Autodesk Inventor part; units mm, degrees
ref_plane "Work Plane1" through (83.5, 0, -139.5) normal (1, 0, 0) x (0, 0, -1)
ref_plane "YZ Plane" through (0, 0, 0) normal (1, 0, 0) x (0, 1, 0)
ref_plane "XZ Plane" through (0, 0, 0) normal (0, 1, 0) x (-1, 0, 0)
sketch "Sketch1" plane through (0, 0, 0) normal (0, 1, 0) x (-1, 0, 0)
  line L0 (-83.5, 139.5) -> (83.5, 139.5)
  line L1 (83.5, 139.5) -> (83.5, -139.5)
  line L2 (83.5, -139.5) -> (-83.5, -139.5)
  line L3 (-83.5, -139.5) -> (-83.5, 139.5)
  line L4 (-83.5, 139.5) -> (83.5, -139.5) construction
  line L5 (83.5, 139.5) -> (-83.5, -139.5) construction
  point P0 (0, 0)
  dimension "d0" = 167
  dimension "d1" = 279
extrude "Extrusion1" add sketch "Sketch1" along normal blind 13.4
sketch "Sketch2" plane through (0, 13.4, 0) normal (0, 1, 0) x (1, 0, 0)
  line L0 (72.25, -115.05) -> (-72.25, -115.05)
  line L1 (-72.25, -115.05) -> (-72.25, 115.05)
  line L2 (-72.25, 115.05) -> (72.25, 115.05)
  line L3 (72.25, 115.05) -> (72.25, -115.05)
  line L4 (72.25, -115.05) -> (-72.25, 115.05) construction
  line L5 (-72.25, -115.05) -> (72.25, 115.05) construction
  point P0 (0, 0)
  dimension "d4" = 144.5
  dimension "d5" = 230.1
extrude "Extrusion2" cut sketch "Sketch2" against normal blind 8.4
sketch "Sketch4" plane through (0, 13.4, 0) normal (0, 1, 0) x (1, 0, 0)
  circle A0 centre (-77.5, -133.5) radius 1.25
  line L0 (-83.5, 139.5) -> (-83.5, -139.5)
  line L1 (-83.5, -139.5) -> (83.5, -139.5)
  circle A1 centre (-77.5, 133.5) radius 1.25
  line L2 (83.5, 139.5) -> (-83.5, 139.5)
  circle A2 centre (77.5, 133.5) radius 1.25
  line L3 (83.5, -139.5) -> (83.5, 139.5)
  circle A3 centre (77.5, -133.5) radius 1.25
  point P0 (0, 0)
  dimension "d16" = 2.5
  dimension "d17" = 6
  dimension "d18" = 6
  dimension "d19" = 2.5
  dimension "d20" = 6
  dimension "d21" = 6
  dimension "d22" = 2.5
  dimension "d23" = 6
  dimension "d24" = 6
  dimension "d25" = 2.5
  dimension "d26" = 6
  dimension "d27" = 6
extrude "Extrusion4" cut sketch "Sketch4" against normal through all contours A0 | A1 | A2 | A3
sketch "Sketch5" plane through (0, 13.4, 0) normal (0, 1, 0) x (1, 0, 0)
  line L0 (-72.25, -115.05) -> (-72.25, 115.05)
  line L1 (72.25, -115.05) -> (-72.25, -115.05)
  line L2 (-77.25, -120.05) -> (-72.25, -120.05)
  line L3 (-72.25, -120.05) -> (-72.25, 120.05)
  line L4 (-72.25, 120.05) -> (-77.25, 120.05)
  line L5 (-77.25, 120.05) -> (-77.25, -120.05)
  line L6 (72.25, 115.05) -> (72.25, -115.05)
  line L7 (77.25, -120.05) -> (72.25, -120.05)
  line L8 (72.25, -120.05) -> (72.25, 120.05)
  line L9 (72.25, 120.05) -> (77.25, 120.05)
  line L10 (77.25, 120.05) -> (77.25, -120.05)
  line L11 (-72.25, 115.05) -> (72.25, 115.05)
  line L12 (72.25, 120.05) -> (-72.25, 120.05)
  line L13 (-72.25, 120.05) -> (-72.25, 115.05)
  line L14 (-72.25, 115.05) -> (72.25, 115.05)
  line L15 (72.25, 115.05) -> (72.25, 120.05)
  line L16 (-72.25, -115.05) -> (72.25, -115.05)
  line L17 (72.25, -115.05) -> (72.25, -120.05)
  line L18 (72.25, -120.05) -> (-72.25, -120.05)
  line L19 (-72.25, -120.05) -> (-72.25, -115.05)
  point P0 (0, 0)
  dimension "d30" = 5
  dimension "d31" = 5
  dimension "d32" = 240.1
  dimension "d33" = 5
  dimension "d34" = 5
  dimension "d35" = 240.1
extrude "Extrusion5" add sketch "Sketch5" along normal blind 10 contours L3 L2 L5 L4 L0 | L1 L8 L18 L3 | L3 L12 L8 L11 | L6 L8 L9 L10 L7
sketch "Sketch7" plane through (0, 0, 0) normal (0, -1, 0) x (1, 0, 0)
  circle A0 centre (-77.5, -133.5) radius 1.25
  circle A1 centre (-77.5, -133.5) radius 1.75
  circle A2 centre (-77.5, 133.5) radius 1.25
  circle A3 centre (-77.5, 133.5) radius 1.75
  circle A4 centre (77.5, 133.5) radius 1.25
  circle A5 centre (77.5, 133.5) radius 1.75
  circle A6 centre (77.5, -133.5) radius 1.25
  circle A7 centre (77.5, -133.5) radius 1.75
  point P0 (0, 0)
  dimension "d42" = 3.5
  dimension "d43" = 3.5
  dimension "d44" = 3.5
  dimension "d45" = 3.5
extrude "Extrusion6" cut sketch "Sketch7" against normal blind 11.4 contours A0 | A1 | A2 | A3 | A4 | A5 | A7
sketch "Sketch8" plane through (83.5, 0, 139.5) normal (1, 0, 0) x (0, 0, -1)
  line L0 (139.5, 0) -> (139.5, 13.4)
  line L1 (0, 13.4) -> (279, 13.4)
sketch "Sketch9" plane through (0, 13.4, 0) normal (0, 1, 0) x (1, 0, 0)
  line L0 (83.5, -139.5) -> (83.5, 139.5)
  line L1 (83.5, 0) -> (77.25, 0)
  line L2 (77.25, 120.05) -> (77.25, -120.05)
  point P0 (0, 0)
sketch "Sketch10" plane through (77.25, 13.4, 120.05) normal (1, 0, 0) x (0, 0, -1)
  line L0 (-19.45, 0) -> (259.55, 0)
  line L1 (120.05, 0) -> (120.05, 10)
  line L2 (0, 10) -> (240.1, 10)
  point P0 (120.05, -13.4)
split_face "Split1"
split_face "Split2"
split_face "Split3"
ref_plane "Work Plane1" through (83.5, 0, -139.5) normal (1, 0, 0) x (0, 0, -1)
sketch "Sketch11" plane through (83.5, 0, -139.5) normal (1, 0, 0) x (0, 0, -1)
  line L0 (0, 0) -> (0, 13.4)
  line L1 (-139.5, 5) -> (-139.5, 23.4)
  line L2 (0, 0) -> (-139.5, 0)
  line L3 (-139.5, 0) -> (-139.5, 23.4)
  line L4 (-139.5, 23.4) -> (0, 23.4)
  line L5 (0, 23.4) -> (0, 0)
  point P0 (-139.5, 0)
extrude "Extrusion7" cut sketch "Sketch11" against normal blind 167.1625
sketch "Sketch12" plane through (83.5, 0, 0) normal (0, 0, -1) x (-1, 0, 0)
  line L0 (0, 0) -> (0, 13.4)
  circle A0 centre (5.625, 6.7) radius 2.375
  line L1 (167, 0) -> (167, 13.4)
  circle A1 centre (161.375, 6.7) radius 2.375
  line L2 (11.25, 5) -> (155.75, 5)
  circle A2 centre (58.5, 2.5) radius 1.375
  circle A3 centre (33.5, 2.5) radius 1.375
  circle A4 centre (108.5, 2.5) radius 1.375
  circle A5 centre (133.5, 2.5) radius 1.375
  point P0 (83.5, 0)
  dimension "d51" = 4.75
  dimension "d53" = 4.75
  dimension "d55" = 2.75
  dimension "d57" = 2.75
  dimension "d59" = 2.75
  dimension "d61" = 2.75
extrude "Extrusion8" add sketch "Sketch12" along normal blind 15
properties part number "Enclosure 2 Bottom" material "ABS Plastic"
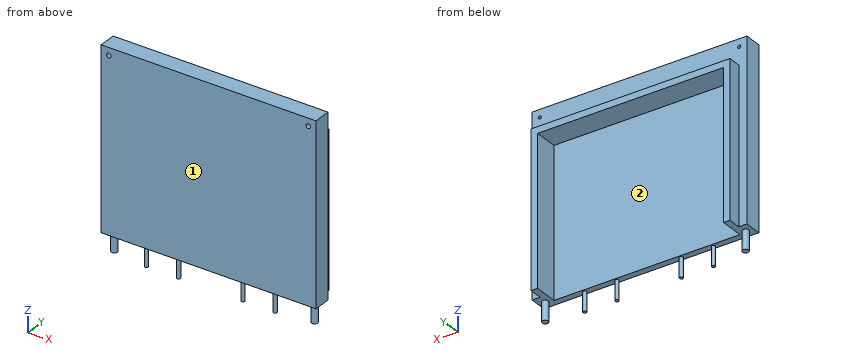
Design review of the part built by this model. Coordinates are the model's own, in mm. Face numbers are marked on the shaded views. Round coordinates to 2 decimals unless told otherwise and drop trailing zeros. Order: outer loops, then holes, each group sorted by start corner. A loop starts at its lowest first (then second) coordinate and runs counter-clockwise, first axis right, second up. Notation, with made-up numbers: M 81.5,32.25 L 119.5,32.25 A12 cw 119.5,51.25 Z; hole C 21,26 d1. An arc over 180 degrees is marked long. Answer as CSV lines item,"result". Start each with the question number.
1) Wall thickness on line 1 along X through (y, z) = (6, 133.5); line 2 along X through (y, z) = (11.9, 133.5); line 3 along X through (y, z) = (12.5, 73): over which ranges is each line inside the solid? List them lowest first. Write a range as [from, to].
2) The part is to be moulded in two halves that separate along X. For the marked faces 1 and 2, say which applies: +X half, -X half, draft (parallel to the pull), parting line (faces both ways), or undercut.
3) Add section A-A (z = -4). Give the boundary of the cut face in (x, y) (3 decimals).
4) Add section B-B (x = 68). Give the boundary of the cut face in (y, z), then the cut area to 3 significant figures.
5) Add section C-C (y = 15.25). Give the boundary of the cut face in (x, z).
6) Add section D-D (z = 91). Give the boundary of the cut face in (x, y).
7) For pin 1 Ø8 at (y, z) = (19, 72.5) entering from +X; pin 2 Ø6 at (x, z) = (-60, 22) entering from +Y; pin 3 Ø3 at (x, y) = (-32.5, 18) entering from +Z, all flat-tipped, find the tip position at first contact; note any pin that passes through.
Resolved:
1,line 1,"[-83.5, -79.25], [-75.75, 75.75], [79.25, 83.5]"
1,line 2,"[-83.5, -78.75], [-76.25, 76.25], [78.75, 83.5]"
1,line 3,"[-83.5, -72.25], [72.25, 83.5]"
2,face 1,"draft"
2,face 2,"undercut"
3,outline,"C -77.875,6.7 d4.75; C -50,2.5 d2.75; C -25,2.5 d2.75; C 25,2.5 d2.75; C 50,2.5 d2.75; C 77.875,6.7 d4.75"
4,outline,"M 0,0 L 5,0 L 5,115.05 L 23.4,115.05 L 23.4,120.05 L 13.4,120.05 L 13.4,139.5 L 0,139.5 Z"
4,area,"953 mm^2"
5,outline,"M -77.25,0 L -72.25,0 L -72.25,115.05 L 72.25,115.05 L 72.25,0 L 77.25,0 L 77.25,120.05 L -77.25,120.05 Z"
6,outline,"M -83.5,0 L 83.5,0 L 83.5,13.4 L 77.25,13.4 L 77.25,23.4 L 72.25,23.4 L 72.25,5 L -72.25,5 L -72.25,23.4 L -77.25,23.4 L -77.25,13.4 L -83.5,13.4 Z"
7,pin 1,"x = 77.25"
7,pin 2,"y = 5"
7,pin 3,"z = 120.05"
